Autodesk Inventor part; units mm, degrees
ref_plane "YZ Plane" through (0, 0, 0) normal (1, 0, 0) x (0, 1, 0)
ref_plane "XZ Plane" through (0, 0, 0) normal (0, 1, 0) x (-1, 0, 0)
ref_plane "XY Plane" through (0, 0, 0) normal (0, 0, 1) x (1, 0, 0)
sketch "スケッチ1" plane through (0, 0, 0) normal (0, 0, 1) x (1, 0, 0)
  circle A0 centre (0, 0) radius 1.5
  circle A1 centre (84.4097, 34) radius 1.5
  line L0 (-20, 50) -> (100, 50)
  line L1 (100, 50) -> (100, -20)
  line L2 (100, -20) -> (-20, -20)
  line L3 (-20, -20) -> (-20, 50)
  dimension "d0" = 3
  dimension "d1" = 3
  dimension "d2" = 91
  dimension "d3" = 34
extrude "押し出し1" add sketch "スケッチ1" along normal blind 3
properties part number "足フレームの代わり"
Input: part model. Units: mm. Frame: model coordinates. Coordinates: 2 decimals unless noted, no trailing zeros. Order: outer loops, then holes, each group sorted by start corner. A loop starts at its lowest first (then second) coordinate and runs counter-clockwise, first axis right, second up. Notation, with made-up numbers: M 16,27.5 L 37,27.5 A26 cw 37,62.5 Z; hole C -28,69 d3. An arc over 180 degrees is marked long. Write item = value, one per line. Start each with the question number.
(1) Section B-B on y = 0. Output: boundary loops of the cut face in (x, z).
(2) Line query: line 1 along Y through (x, z) = (0, 0.95); line 2 along X through (y, z) = (33.5, 0.85). Output: solid intervals per line, ascending. Write a range as [from, to].
(3) Section A-A on x = 0. Output: boundary loops of the cut face in (y, z).
(4) Pull-direction query (X, two-part tool) for faces 1 (the cylindrical face through (-1.5, -0.07, 1.48)), 2 (the flat face through (39, 15, 0)), 3 (the flat face through (-20, 15, 1)); classes: released by +X, released by -X, zero draft, split by the parting line, or undercut.
Result set:
q1.outline = M -20,0 L -1.5,0 L -1.5,3 L -20,3 Z; M 1.5,0 L 100,0 L 100,3 L 1.5,3 Z
q2.line_1 = [-20, -1.5], [1.5, 50]
q2.line_2 = [-20, 83], [85.82, 100]
q3.outline = M -20,0 L -1.5,0 L -1.5,3 L -20,3 Z; M 1.5,0 L 50,0 L 50,3 L 1.5,3 Z
q4.face_1 = undercut
q4.face_2 = zero draft
q4.face_3 = released by -X
